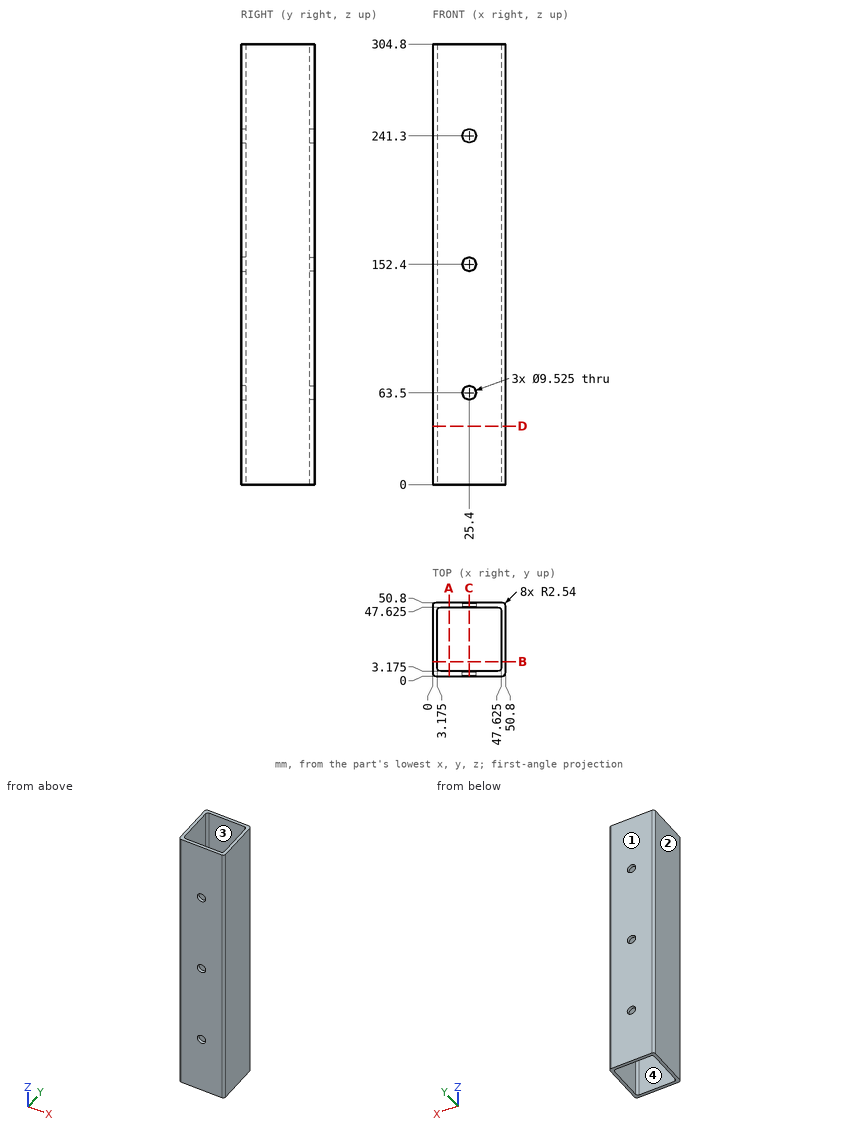
Verification items for this drawing (mm, ordinates from the low corner). Coordinates: 2 decimals unless noted, no trailing zeros. Write each loop counter-clockwise with the first axis right and the second up, starting at its lowest first coordinate (ties: lowest second). Pieces come first, ordered by that corner, then holes. Notation, with made-up numbers: M -30,-2 L -26,-2 A12 ccw -26,4 Z; hole C 60,44 d11. An arc over 180 degrees is marked long. Answer as a JSON object with one key per item and string values. Group by question number.
(1) Cross-section at A-A, the plane x = 11.5. Record the cut outline in (y, z) (3 decimals), and give its area (3 significant figures).
(2) Release check for a two-part mould opening along Y. For the marked faces 1, 2, 3 and 4 record: +Y half, -Y half, draft (parallel to the pull), parting line (faces both ways), or undercut.
(3) Material ranges on line 1 (Z direction, x = 25, y = 1); line 2 (Y direction, x = 40, z = 63) (3 decimals), recorded low to high.
(4) Cross-section at D-D, the plane z = 40.5. Record the cut outline in (x, y) (3 decimals).
(5) Cross-section at C-C, the plane x = 25.4. State how many separate pieces and enclosed holes the cut face has, and give its area (3 significant figures).
Reply:
{
 "1": {"outline": "M 0,0 L 3.175,0 L 3.175,304.8 L 0,304.8 Z; M 47.625,0 L 50.8,0 L 50.8,304.8 L 47.625,304.8 Z", "area": "1,940 mm²"},
 "2": {"face 1": "+Y half", "face 2": "draft", "face 3": "undercut", "face 4": "undercut"},
 "3": {"line 1": "0 to 58.75, 68.25 to 147.65, 157.15 to 236.55, 246.05 to 304.8", "line 2": "0 to 3.175, 47.625 to 50.8"},
 "4": {"outline": "M 0,2.54 A2.54 ccw 2.54,0 L 48.26,0 A2.54 ccw 50.8,2.54 L 50.8,48.26 A2.54 ccw 48.26,50.8 L 2.54,50.8 A2.54 ccw 0,48.26 Z; hole M 3.175,5.715 A2.54 ccw 5.715,3.175 L 45.085,3.175 A2.54 ccw 47.625,5.715 L 47.625,45.085 A2.54 ccw 45.085,47.625 L 5.715,47.625 A2.54 ccw 3.175,45.085 Z"},
 "5": {"separate pieces": "8", "enclosed holes": "0", "area": "1,750 mm²"}
}
